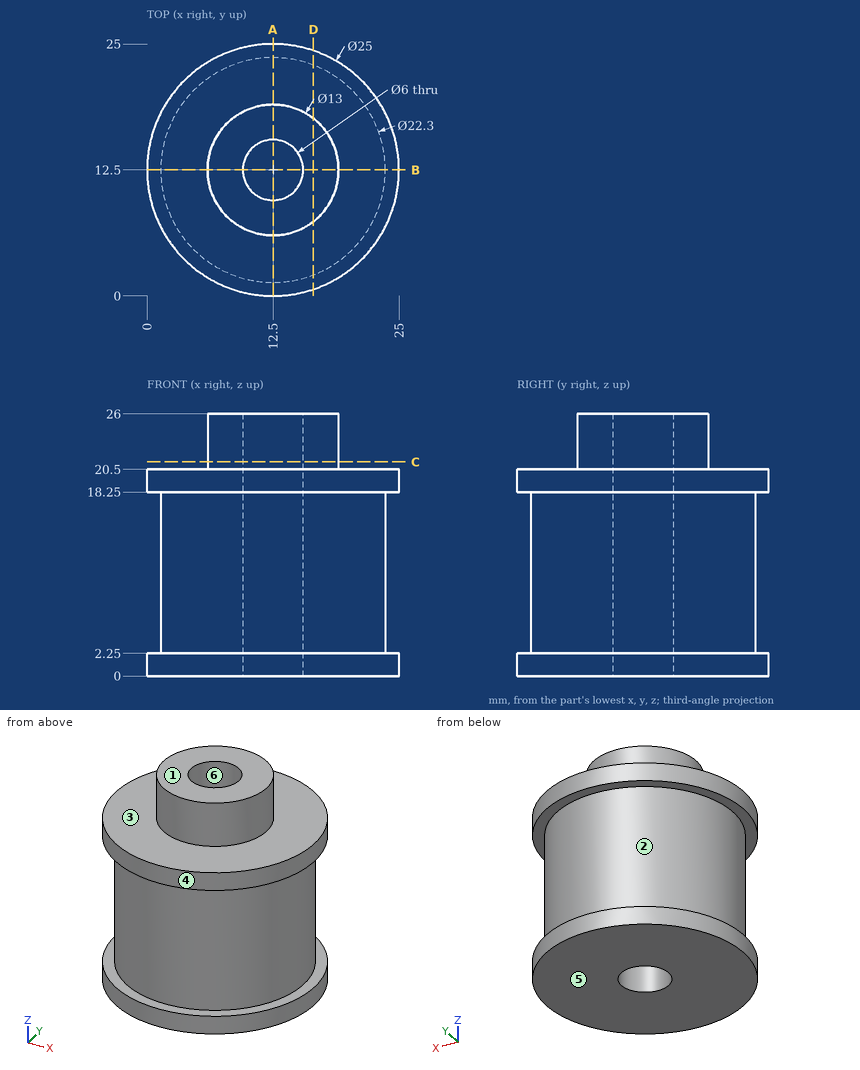
For this review, use the dimensioned drawing (mm, ordinates from the lowest corner) and the shaded views. A direction names the side the tool comes from. Coordinates: 2 decimals unless noted, no trailing zeros. Order: outer loops, then holes, each group sorted by start corner. A loop starts at its lowest first (then second) coordinate and runs counter-clockwise, first axis right, second up. Notation, with made-up numbers: (86, 78.5) - (126, 78.5) arc R10 ccw to (126, 93.5) - close; hole circle Ø11 at (42, -4.5). An arc over 180 degrees is marked (long way). Answer in a Markdown table with one row per item.
(1) Clearance check with flat-ended pins moving along their axes: pin 1 (6 mm diameter, centred on y = 16.5, z = 11, fed in from +X); pin 2 (1 mm diameter, centred on y = 4.5, z = 14, fed in from +X); pin 3 (4 mm diameter, centred on x = 21.5, y = 20, fed in from +Z). State where each tip first meets the part, or that it passes through.
Checked values:
| item | result |
|---|---|
| pin 1 | x = 23.61 |
| pin 2 | x = 20.75 |
| pin 3 | z = 20.5 |
(2) Consider section C-C on z = 21.25. State the section outline as (x, y) points.
Checked values:
| item | result |
|---|---|
| outline | circle Ø13 at (12.5, 12.5); hole circle Ø6 at (12.5, 12.5) |
(3) The part is to be moulded in two halves that separate along Y. For the marked faces 4, 5 and 6, say which applies: released by +Y, released by -Y, zero draft, split by the parting line, or undercut.
Checked values:
| item | result |
|---|---|
| face 4 | split by the parting line |
| face 5 | zero draft |
| face 6 | undercut |
(4) For the marked faces 1, 2 and 3, list the 3-axis set-ups (+Z, -Z, +X, -X, +Y, -Y) from which the entire face can be reached by the end or side of a thin tool; tool diameter is ignored.
Checked values:
| item | result |
|---|---|
| face 1 | +Z, +X, -X, +Y, -Y |
| face 2 | none |
| face 3 | +Z |
(5) Consider section A-A on x = 12.5. State the section outline as (y, z) points.
Checked values:
| item | result |
|---|---|
| outline | (0, 0) - (9.5, 0) - (9.5, 26) - (6, 26) - (6, 20.5) - (0, 20.5) - (0, 18.25) - (1.35, 18.25) - (1.35, 2.25) - (0, 2.25) - close; (15.5, 0) - (25, 0) - (25, 2.25) - (23.65, 2.25) - (23.65, 18.25) - (25, 18.25) - (25, 20.5) - (19, 20.5) - (19, 26) - (15.5, 26) - close |
(6) Wall thickness on line 1 along Y through (x, z) = (12.5, 16); line 2 along Y through (x, z) = (12.5, 21.75); line 3 along Z through (x, y) = (19.5, 10): over which ranges is each line inside the solid? List them lowest first. Write a range as from..to.
Checked values:
| item | result |
|---|---|
| line 1 | 1.35..9.5, 15.5..23.65 |
| line 2 | 6..9.5, 15.5..19 |
| line 3 | 0..20.5 |
(7) Consider section D-D on x = 16.5. State the section outline as (y, z) points.
Checked values:
| item | result |
|---|---|
| outline | (0.66, 0) - (24.34, 0) - (24.34, 2.25) - (22.91, 2.25) - (22.91, 18.25) - (24.34, 18.25) - (24.34, 20.5) - (17.62, 20.5) - (17.62, 26) - (7.38, 26) - (7.38, 20.5) - (0.66, 20.5) - (0.66, 18.25) - (2.09, 18.25) - (2.09, 2.25) - (0.66, 2.25) - close |
